```python
from build123d import *

# Parameters (mm, degrees)
SKETCH1_R      = 2.5527
EXTRUDE1_DEPTH = 82.55


with BuildPart() as part:
    # Sketch1 → Extrude1 (new body)
    with BuildSketch(Plane.XY):
        with BuildLine():
            Line((3.238504286, -11.455400345), (3.238504286, -11.49073383))
            ThreePointArc((3.238504286, -11.49073383), (3.509397472, -12.161218003), (4.170019162, -12.455345741))
            Line((4.170019162, -12.455345741), (11.176001705, -12.7))
            ThreePointArc((11.176001705, -12.7), (12.253632411, -12.253630746), (12.700001664, -11.17600004))
            Line((12.700001664, -11.17600004), (12.455347406, -4.170014669))
            ThreePointArc((12.455347406, -4.170014669), (12.16121968, -3.509392954), (11.490735494, -3.238499755))
            Line((11.490735494, -3.238499755), (11.455402009, -3.238499755))
            ThreePointArc((11.455402009, -3.238499755), (10.772902626, -3.521200256), (10.490202125, -4.20369964))
            Line((10.490202125, -4.20369964), (10.490202125, -6.352134987))
            ThreePointArc((10.490202125, -6.352134987), (9.831646779, -7.337732713), (8.669054992, -7.106478829))
            Line((8.669054992, -7.106478829), (4.820959759, -3.258383596))
            ThreePointArc((4.820959759, -3.258383596), (4.589705874, -2.912287699), (4.508500309, -2.504039754))
            Line((4.508500309, -2.504039754), (4.508500309, 2.504040946))
            ThreePointArc((4.508500309, 2.504040946), (4.589705874, 2.912288891), (4.820959759, 3.258384788))
            Line((4.820959759, 3.258384788), (8.669054992, 7.106480021))
            ThreePointArc((8.669054992, 7.106480021), (9.831646779, 7.337733906), (10.490202125, 6.35213618))
            Line((10.490202125, 6.35213618), (10.490202125, 4.203700832))
            ThreePointArc((10.490202125, 4.203700832), (10.772902626, 3.521201448), (11.455402009, 3.238500947))
            Line((11.455402009, 3.238500947), (11.490735494, 3.238500947))
            ThreePointArc((11.490735494, 3.238500947), (12.161219667, 3.509394133), (12.455347406, 4.170015823))
            Line((12.455347406, 4.170015823), (12.700001664, 11.176000039))
            ThreePointArc((12.700001664, 11.176000039), (12.253632411, 12.253630745), (11.176001705, 12.699999999))
            Line((11.176001705, 12.699999999), (4.170019162, 12.455345462))
            ThreePointArc((4.170019162, 12.455345462), (3.509397447, 12.161217736), (3.238504248, 11.49073355))
            Line((3.238504248, 11.49073355), (3.238504248, 11.455400065))
            ThreePointArc((3.238504248, 11.455400065), (3.521204749, 10.772900682), (4.203704132, 10.490200181))
            Line((4.203704132, 10.490200181), (6.35213948, 10.490200181))
            ThreePointArc((6.35213948, 10.490200181), (7.337737205, 9.831644835), (7.106483322, 8.669053049))
            Line((7.106483322, 8.669053049), (3.258388088, 4.820957816))
            ThreePointArc((3.258388088, 4.820957816), (2.912292192, 4.589703931), (2.504044247, 4.508498366))
            Line((2.504044247, 4.508498366), (-2.504036453, 4.508498366))
            ThreePointArc((-2.504036453, 4.508498366), (-2.912284398, 4.589703931), (-3.258380295, 4.820957816))
            Line((-3.258380295, 4.820957816), (-7.106475528, 8.669053049))
            ThreePointArc((-7.106475528, 8.669053049), (-7.337729412, 9.831644836), (-6.352131686, 10.490200182))
            Line((-6.352131686, 10.490200182), (-4.203696339, 10.490200182))
            ThreePointArc((-4.203696339, 10.490200182), (-3.521196955, 10.772900683), (-3.238496454, 11.455400067))
            Line((-3.238496454, 11.455400067), (-3.238496454, 11.490733551))
            ThreePointArc((-3.238496454, 11.490733551), (-3.50938964, 12.161217724), (-4.17001133, 12.455345462))
            Line((-4.17001133, 12.455345462), (-11.175998375, 12.699999999))
            ThreePointArc((-11.175998375, 12.699999999), (-12.253629081, 12.253630745), (-12.699998335, 11.176000039))
            Line((-12.699998335, 11.176000039), (-12.455343798, 4.170015823))
            ThreePointArc((-12.455343798, 4.170015823), (-12.161216073, 3.509394108), (-11.490731887, 3.238500909))
            Line((-11.490731887, 3.238500909), (-11.455398403, 3.238500909))
            ThreePointArc((-11.455398403, 3.238500909), (-10.772899019, 3.52120141), (-10.490198518, 4.203700793))
            Line((-10.490198518, 4.203700793), (-10.490198518, 6.352136141))
            ThreePointArc((-10.490198518, 6.352136141), (-9.831643172, 7.337733867), (-8.669051385, 7.106479983))
            Line((-8.669051385, 7.106479983), (-4.820956152, 3.258384749))
            ThreePointArc((-4.820956152, 3.258384749), (-4.589702267, 2.912288853), (-4.508496702, 2.504040908))
            Line((-4.508496702, 2.504040908), (-4.508496702, -2.504039793))
            ThreePointArc((-4.508496702, -2.504039793), (-4.589702267, -2.912287738), (-4.820956152, -3.258383634))
            Line((-4.820956152, -3.258383634), (-8.669051385, -7.106478867))
            ThreePointArc((-8.669051385, -7.106478867), (-9.831643172, -7.337732752), (-10.490198518, -6.352135026))
            Line((-10.490198518, -6.352135026), (-10.490198518, -4.203699678))
            ThreePointArc((-10.490198518, -4.203699678), (-10.772899019, -3.521200294), (-11.455398403, -3.238499793))
            Line((-11.455398403, -3.238499793), (-11.490731887, -3.238499793))
            ThreePointArc((-11.490731887, -3.238499793), (-12.16121606, -3.509392979), (-12.455343798, -4.170014669))
            Line((-12.455343798, -4.170014669), (-12.699998335, -11.17600004))
            ThreePointArc((-12.699998335, -11.17600004), (-12.253629081, -12.253630746), (-11.175998375, -12.7))
            Line((-11.175998375, -12.7), (-4.17001133, -12.455345741))
            ThreePointArc((-4.17001133, -12.455345741), (-3.509389615, -12.161218016), (-3.238496416, -11.49073383))
            Line((-3.238496416, -11.49073383), (-3.238496416, -11.455400345))
            ThreePointArc((-3.238496416, -11.455400345), (-3.521196917, -10.772900961), (-4.2036963, -10.49020046))
            Line((-4.2036963, -10.49020046), (-6.352131648, -10.49020046))
            ThreePointArc((-6.352131648, -10.49020046), (-7.337729374, -9.831645114), (-7.106475489, -8.669053328))
            Line((-7.106475489, -8.669053328), (-3.258380256, -4.820958094))
            ThreePointArc((-3.258380256, -4.820958094), (-2.91228436, -4.58970421), (-2.504036415, -4.508498645))
            Line((-2.504036415, -4.508498645), (2.504044285, -4.508498645))
            ThreePointArc((2.504044285, -4.508498645), (2.91229223, -4.58970421), (3.258388127, -4.820958094))
            Line((3.258388127, -4.820958094), (7.10648336, -8.669053328))
            ThreePointArc((7.10648336, -8.669053328), (7.337737245, -9.831645114), (6.352139519, -10.49020046))
            Line((6.352139519, -10.49020046), (4.203704171, -10.49020046))
            ThreePointArc((4.203704171, -10.49020046), (3.521204787, -10.772900961), (3.238504286, -11.455400345))
        make_face()
        Circle(SKETCH1_R, mode=Mode.SUBTRACT)
    extrude(amount=EXTRUDE1_DEPTH)


solid = part.part
```
The listing builds one solid part. Answer for the finished solid, in the listing's coordinates (mm). Give positions to 0.01 mm unless a question says otherwise; leave off trailing zeros. Order: outer loops, then holes, each group sorted by start corner. A loop starts at its lowest first (then second) coordinate and runs counter-clockwise, first axis right, second up. Notation, with made-up numbers: (-4.5, -39) - (45.5, -39) arc R32 cw to (45.5, 0) - close; hole circle Ø2 at (12, -13). An arc over 180 degrees is marked (long way). Use one line per item in the form item = value. Start each with the question number.
(1) Flat-ended cylindrical pins translate along their axes: pin 1 Ø2.5 at (x, z) = (-0.5, 27.5) entering from +Y; pin 2 Ø1.5 at (x, z) = (-0.5, 22) entering from -Y; pin 3 Ø10 at (y, z) = (-5.5, 21.5) entering from +X. Find the tip coordinate at first contact, or state that the pin passes through.
(2) The mould has two halves that part along Y. Classify faces 1 (the flat face through (4.509, 0, 41)), 2 (the flat face through (-3, 0, 0)), 3 (the flat face through (0, 4.508, 41)), 4 (the cylindrical face through (-7.33, -9.85, 40.7)): released by +Y, released by -Y, zero draft, split by the parting line, or undercut.
(3) A cutting plane is placed at A-A, the plane x = 0. Write down the section's boundary in (y, z).
(4) Consider line 1 (X direction, y = -0.5, z = 71.5); line 2 (Y direction, x = -6, z = 21); line 3 (Y direction, x = 0, z = 8.5). Determine where each line is inside the solid, lowest interval first. Write a range as from..to.
Ans:
q1.pin_1 = 4.51
q1.pin_2 = -4.51
q1.pin_3 = 12.68
q2.face_1 = undercut
q2.face_2 = zero draft
q2.face_3 = released by +Y
q2.face_4 = undercut
q3.outline = (-4.51, 0) - (-2.55, 0) - (-2.55, 82.55) - (-4.51, 82.55) - close; (2.55, 0) - (4.51, 0) - (4.51, 82.55) - (2.55, 82.55) - close
q4.line_1 = -4.51..-2.5, 2.5..4.51
q4.line_2 = -12.52..-10.49, -7.56..-4.44, 4.44..7.56, 10.49..12.52
q4.line_3 = -4.51..-2.55, 2.55..4.51
